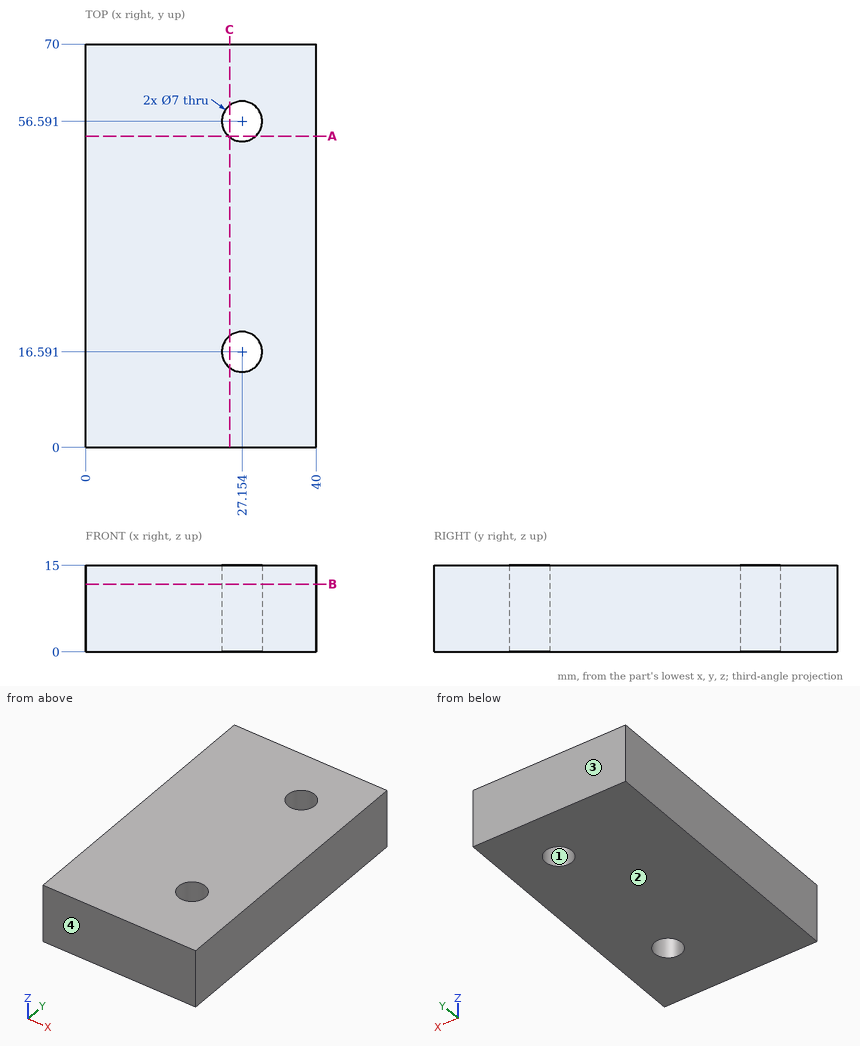
Study the drawing (mm; zero at the part's minimum x, y, z) and answer. Coordinates: 2 decimals unless noted, no trailing zeros. Loops run counter-clockwise (first coordinate to the right, second up) from the corner with the lowest first, then second, coordinate; pieces in that order, holes last. Notation, with made-up numbers: (7.5, 30.25) -> (30.5, 30.25) arc R8 cw to (30.5, 41.25) -> close; hole circle Ø7 at (59.25, 17.25). An arc over 180 degrees is marked (long way). Write each question's results on one line, items separated by ' | '. Start each with the question number.
1) Find section A-A on y = 54. Determine the outline of the cut face in (x, z), then the cut area to 3 significant figures.
2) Consider line 1 along Y through (x, z) = (26.5, 9.5); line 2 along X through (y, z) = (16, 1.25). Determine where each line is inside the solid, lowest interval first.
3) Find section B-B on z = 11.75. Determine the outline of the cut face in (x, y), then the cut area to 3 significant figures.
4) The mould has two halves that part along Y. Classify the marked faces 1, 2, 3 and 4: pulls with the +Y half, pulls with the -Y half, needs draft (parallel to the pull), parting line crosses it, or undercut.
5) Find section C-C on x = 25. Determine the outline of the cut face in (y, z).
Response values:
1) outline: (0, 0) -> (24.8, 0) -> (24.8, 15) -> (0, 15) -> close; (29.51, 0) -> (40, 0) -> (40, 15) -> (29.51, 15) -> close | area: 529 mm^2
2) line 1: y = 0 to 13.15, 20.03 to 53.15, 60.03 to 70 | line 2: x = 0 to 23.7, 30.6 to 40
3) outline: (0, 0) -> (40, 0) -> (40, 70) -> (0, 70) -> close; hole circle Ø7 at (27.15, 16.59); hole circle Ø7 at (27.15, 56.59) | area: 2,720 mm^2
4) face 1: undercut | face 2: needs draft | face 3: pulls with the +Y half | face 4: pulls with the -Y half
5) outline: (0, 0) -> (13.83, 0) -> (13.83, 15) -> (0, 15) -> close; (19.35, 0) -> (53.83, 0) -> (53.83, 15) -> (19.35, 15) -> close; (59.35, 0) -> (70, 0) -> (70, 15) -> (59.35, 15) -> close
